Autodesk Inventor part; units mm, degrees
ref_plane "YZ Plane" through (0, 0, 0) normal (1, 0, 0) x (0, 1, 0)
ref_plane "XZ Plane" through (0, 0, 0) normal (0, 1, 0) x (-1, 0, 0)
sketch "Boceto1" plane through (0, 0, 0) normal (0, 0, 1) x (1, 0, 0)
  arc A0 (0, 5) -> (0, -5) centre (0, 0) ccw
  line L0 (0, 5) -> (0, -5)
revolve "Revolución1" add sketch "Boceto1" angle 360 about axis through (0, 5, 0) along (0, -1, 0)
ref_plane "Plano de trabajo1" through (0, 0, 5) normal (0, 0, 1) x (1, 0, 0)
sketch "Boceto2" plane through (0, 0, 5) normal (0, 0, 1) x (1, 0, 0)
  line L0 (-2, -10) -> (2, -10)
  line L1 (2, -10) -> (2, 10)
  line L2 (2, 10) -> (-2, 10)
  line L3 (-2, 10) -> (-2, -10)
  line L4 (-2, -10) -> (2, 10) construction
  line L5 (2, -10) -> (-2, 10) construction
  point P0 (0, 0)
  dimension "d3" = 4
  dimension "d4" = 20
extrude "Extrusión1" add sketch "Boceto2" against normal blind 2
sketch "Boceto3" plane through (0, 0, 5) normal (0, 0, 1) x (1, 0, 0)
  point P0 (0, 0)
  point P1 (0, 7.5)
  point P2 (0, -7.5)
hole "Agujero1" at (0, 7.5, 5) at (0, -7.5, 5) direction (0, 0, -1) diameter 3.175 end through all
properties part number "Rueda trasera"
Geometry check sheet. Reference: the model listing, model coordinates, mm. A direction names the side the tool comes from. Give positions to 0.01 mm unless a question says otherwise; leave off trailing zeros. Write each loop counter-clockwise with the first axis right and the second up, starting at its lowest first coordinate (ties: lowest second). Pieces come first, ordered by that corner, then holes.
1) Release check for a two-part mould opening along Y. For faces 1 (the cylindrical face through (-0.477, -9.014, 3.986)), 2 (the flat face through (0, -10, 4)), 3 (the cylindrical face through (-0.477, 5.986, 3.986)), 4 (the flat face through (1, 6, 3)) record: pulls with the +Y half, pulls with the -Y half, needs draft (parallel to the pull), parting line crosses it, or undercut.
2) Section check A-A, the plane y = 7.5. Record the boundary of the cut face in (x, z).
3) Section check B-B, the plane x = 0. Record the boundary of the cut face in (y, z), and give its area (3 significant figures).
4) Access from +Z, -Z, +X, -X, +Y, -Y to the whole of each face (thin tool, end or side, straight path). Record for faces 5 (the flat face through (0, 10, 4)), 6 (the flat face through (2, -2.4, 4.2)), 7 (the flat face through (-2, 2.4, 4.2)).
5) Gauge pin test, flat ends, axial feed: pin 1 (4.5 mm diameter, centred on x = -0.5, y = -6, fed in from -Z); pin 2 (1 mm diameter, centred on x = -2, y = 0.5, fed in from -Z); pin 3 (3 mm diameter, centred on y = -2.5, z = -0.5, fed in from -X). Record the tip position at first contact, or that the pin passes through.
6) Material ranges on L1, parallel to Y at x = 0, z = 4; L2, parallel to X at y = 7.5, z = 4.6; L3, parallel to Z at x = -1.25, y = -5.75, recorded low to high.
7) Section check D-D, the plane x = -1.25. Record the boundary of the cut face in (y, z), and give its area (4 significant figures).
8) Section check C-C, the plane z = -3. Record the boundary of the cut face in (x, y), and give its area (3 significant figures).
Computed:
1. face 1: undercut
1. face 2: pulls with the -Y half
1. face 3: undercut
1. face 4: needs draft
2. outline: (-2, 3) - (-1.59, 3) - (-1.59, 5) - (-2, 5) - close; (1.59, 3) - (2, 3) - (2, 5) - (1.59, 5) - close
3. outline: (-10, 3) - (-9.09, 3) - (-9.09, 5) - (-10, 5) - close; (-5.91, 3) - (-4, 3) arc R5 ccw (long way) to (4, 3) - (5.91, 3) - (5.91, 5) - (-5.91, 5) - close; (9.09, 3) - (10, 3) - (10, 5) - (9.09, 5) - close
3. area: 94.7 mm2
4. face 5: +Z, -Z, +X, -X, +Y
4. face 6: +Z, +X
4. face 7: +Z, -X
5. pin 1: stops at z = -3.28
5. pin 2: stops at z = -4.75
5. pin 3: stops at x = -4.89
6. L1: y = -10 to -9.09, -5.91 to 5.91, 9.09 to 10
6. L2: x = -2 to -1.59, 1.59 to 2
6. L3: z = 3 to 5
7. outline: (-10, 3) - (-8.48, 3) - (-8.48, 5) - (-10, 5) - close; (-6.52, 3) - (-3.8, 3) arc R4.84 ccw (long way) to (3.8, 3) - (6.52, 3) - (6.52, 5) - (-6.52, 5) - close; (8.48, 3) - (10, 3) - (10, 5) - (8.48, 5) - close
7. area: 96.05 mm2
8. outline: circle Ø8 at (0, 0)
8. area: 50.3 mm2
